from build123d import *

# Parameters (mm, degrees)
SKETCH1_W           = 12.7
SKETCH1_H           = 12.7
BOSS_EXTRUDE1_DEPTH = 2.54
FILLET1_R           = 0.635
SHELL1_START        = 0.635
SHELL1_OUTLINE_W    = 1.905
SHELL1_OUTLINE_H    = 11.43
SHELL1_DEPTH        = 11.43
SKETCH2_R           = 2.54
BOSS_EXTRUDE2_DEPTH = 1.905
BOSS_EXTRUDE4_DEPTH = 0.00254


# Read off the part's stored shape, not the designer's step: Shell1
with BuildPart() as part:
    # Sketch1 → Boss-Extrude1 (new body)
    with BuildSketch(Plane(origin=(0, 0, 0), x_dir=(1, 0, 0), z_dir=(0, 1, 0))):
        with Locations((6.35, 6.35)):
            Rectangle(SKETCH1_W, SKETCH1_H)
    extrude(amount=BOSS_EXTRUDE1_DEPTH)

    # Fillet1
    fillet1_edges = [part.edges().sort_by_distance(p)[0] for p in [
        (0, 1.27, -12.7),
        (12.7, 1.27, -12.7),
        (12.7, 1.27, 0),
        (0, 1.27, 0),
    ]]
    fillet(fillet1_edges, radius=FILLET1_R)

    # Shell1 outline → Shell1 (cut)
    with BuildSketch(Plane.YZ.offset(SHELL1_START)):
        with Locations((0.9525, -6.35)):
            Rectangle(SHELL1_OUTLINE_W, SHELL1_OUTLINE_H)
    extrude(amount=SHELL1_DEPTH, mode=Mode.SUBTRACT)

    # Sketch2 → Boss-Extrude2 (add)
    with BuildSketch(Plane(origin=(0, 1.905, 0), x_dir=(-1, 0, 0), z_dir=(0, -1, 0))):
        with Locations(Location((-6.35, 6.35, 0), (0, 0, 270))):
            Circle(SKETCH2_R)
    extrude(amount=BOSS_EXTRUDE2_DEPTH)

    # Sketch4 → Boss-Extrude4 (add)
    # profile 1 of 2: a face of its own
    with BuildSketch(Plane(origin=(0, 2.54, 0), x_dir=(1, 0, 0), z_dir=(0, 1, 0))):
        with BuildLine():
            Line((6.456138622, 5.974210256), (6.960500601, 5.71853117))
            Line((6.960500601, 5.71853117), (6.407165264, 4.630941026))
            add(Edge.make_bspline(
                [(6.407165264, 4.630941026), (6.439855797, 4.630094651), (6.504245162, 4.628427578), (6.598981047, 4.614954014), (6.689550316, 4.591661453), (6.776866176, 4.560787227), (6.859861273, 4.519322834), (6.939872289, 4.469998775), (7.014829299, 4.40984278), (7.086451002, 4.34319313), (7.151576249, 4.269354895), (7.20814904, 4.190013367), (7.257451228, 4.107098934), (7.295776765, 4.018756598), (7.32669142, 3.926450736), (7.348997703, 3.82981236), (7.361724062, 3.728561626), (7.363478603, 3.659777417), (7.364371795, 3.624761138)],
                knots=[0, 0, 0, 0, 1.013260694, 1.995783107, 2.958651975, 3.908806537, 4.861209129, 5.829647963, 6.817170299, 7.835534541, 8.860094905, 9.863329007, 10.853101798, 11.844815043, 12.84250023, 13.867713965, 14.914507806, 16, 16, 16, 16], degree=3))
            add(Edge.make_bspline(
                [(7.364371795, 3.624761138), (7.3635348, 3.591007569), (7.361880421, 3.524291238), (7.348204784, 3.426301914), (7.326104237, 3.332286889), (7.294518118, 3.242433922), (7.254369605, 3.156303809), (7.205270694, 3.073947091), (7.146814203, 2.995979194), (7.080510488, 2.922814401), (7.008029089, 2.856124152), (6.931629747, 2.796845977), (6.850665063, 2.747879955), (6.766665364, 2.706527002), (6.678084165, 2.675668741), (6.586247088, 2.652376099), (6.490457705, 2.638935234), (6.425438326, 2.63724503), (6.392536859, 2.636389744)],
                knots=[0, 0, 0, 0, 1.049934834, 2.075270938, 3.072134561, 4.05064612, 5.033440221, 6.024524368, 7.028587226, 8.060776465, 9.092543989, 10.090062252, 11.064205434, 12.031961459, 12.998029633, 13.977230324, 14.976426867, 16, 16, 16, 16], degree=3))
            add(Edge.make_bspline(
                [(6.392536859, 2.636389744), (6.358131923, 2.637091632), (6.290479272, 2.6384718), (6.191486511, 2.653926046), (6.096543934, 2.677190259), (6.006185133, 2.710407602), (5.919848194, 2.752703587), (5.838549577, 2.805040616), (5.761604456, 2.866841549), (5.689833178, 2.936715965), (5.625172604, 3.013253826), (5.567500777, 3.092720054), (5.518710337, 3.175239347), (5.479215613, 3.260723478), (5.448400913, 3.348900047), (5.426960167, 3.439936406), (5.412989542, 3.53359108), (5.411351805, 3.597150442), (5.410525641, 3.629213261)],
                knots=[0, 0, 0, 0, 1.063775006, 2.091769615, 3.092589432, 4.084662827, 5.064601646, 6.061867366, 7.070035304, 8.113879863, 9.156342271, 10.166834137, 11.149076039, 12.117706134, 13.076241869, 14.034148791, 15.008317125, 16, 16, 16, 16], degree=3))
            add(Edge.make_bspline(
                [(5.410525641, 3.629213261), (5.41096217, 3.654042164), (5.411837658, 3.703838176), (5.420635786, 3.778404999), (5.434012031, 3.853167552), (5.449516851, 3.916254562), (5.465482147, 3.969601232), (5.481551341, 4.014747076), (5.501465566, 4.064849092), (5.524230475, 4.12003522), (5.550561942, 4.180239071), (5.580322415, 4.245296544), (5.613585986, 4.315700304), (5.637307493, 4.364056786), (5.649668269, 4.389254327)],
                knots=[0, 0, 0, 0, 1.110454016, 2.227089276, 3.35462975, 4.507227546, 5.131400587, 5.845402449, 6.650387134, 7.543487832, 8.516250726, 9.590168902, 10.744287919, 12, 12, 12, 12], degree=3))
            Line((5.649668269, 4.389254327), (6.456138622, 5.974210256))
        make_face()
        with BuildLine():
            add(Edge.make_bspline(
                [(6.379816506, 4.101774359), (6.352472323, 4.100520139), (6.298963346, 4.098065795), (6.222881583, 4.072362713), (6.153512277, 4.032040974), (6.093382105, 3.975885155), (6.043088748, 3.908776745), (6.006131425, 3.832230641), (5.983899541, 3.747268327), (5.981589791, 3.687864094), (5.980397436, 3.657198037)],
                knots=[0, 0, 0, 0, 0.981744412, 1.921144944, 2.858899012, 3.85339082, 4.86292663, 5.863643845, 6.897155691, 8, 8, 8, 8], degree=3))
            add(Edge.make_bspline(
                [(5.980397436, 3.657198037), (5.981809222, 3.626521768), (5.984555239, 3.566854373), (6.007623071, 3.481083067), (6.045392269, 3.402798689), (6.098361161, 3.334800948), (6.160545878, 3.278357558), (6.229501354, 3.236614972), (6.304077387, 3.210971132), (6.35566345, 3.207842243), (6.381724559, 3.206261538)],
                knots=[0, 0, 0, 0, 1.098279937, 2.136227893, 3.159405121, 4.194678092, 5.206500211, 6.154139736, 7.067477469, 8, 8, 8, 8], degree=3))
            add(Edge.make_bspline(
                [(6.381724559, 3.206261538), (6.409248036, 3.207870396), (6.463226355, 3.211025646), (6.54109362, 3.23559044), (6.612225834, 3.276633701), (6.67512047, 3.332896382), (6.729145767, 3.400118178), (6.766525816, 3.478862388), (6.790660084, 3.565252761), (6.79319133, 3.625862449), (6.7945, 3.657198037)],
                knots=[0, 0, 0, 0, 0.96921794, 1.900804717, 2.848419905, 3.844199796, 4.861108892, 5.867439427, 6.897452859, 8, 8, 8, 8], degree=3))
            add(Edge.make_bspline(
                [(6.7945, 3.657198037), (6.793009186, 3.687846189), (6.79012205, 3.747199913), (6.768436237, 3.832560256), (6.729717682, 3.908811323), (6.678286397, 3.976162168), (6.616086864, 4.032292947), (6.543941256, 4.072680703), (6.464383952, 4.098020258), (6.408416654, 4.100504747), (6.379816506, 4.101774359)],
                knots=[0, 0, 0, 0, 1.083229974, 2.097801324, 3.086792542, 4.086858909, 5.079819718, 6.026392613, 6.991456328, 8, 8, 8, 8], degree=3))
        make_face(mode=Mode.SUBTRACT)
    # profile 2 of 2: a face of its own
    with BuildSketch(Plane(origin=(0, 2.54, 0), x_dir=(1, 0, 0), z_dir=(0, 1, 0))):
        Polygon((6.235008013, 10.541), (6.653507612, 10.541), (7.542660256, 8.180102564), (7.026213942, 8.180102564), (6.443621795, 9.726897436), (5.86039363, 8.180102564), (5.344583333, 8.180102564), align=None)
    extrude(amount=BOSS_EXTRUDE4_DEPTH)


solid = part.part
Design review of the part built by this model. Coordinates are the model's own, in mm. A direction names the side the tool comes from. Give positions to 0.01 mm unless a question says otherwise; leave off trailing zeros. Loops run counter-clockwise (first coordinate to the right, second up) from the corner with the lowest first, then second, coordinate; pieces in that order, holes last. Notation, with made-up numbers: M 11.25,17.25 L 58.25,17.25 A23 cw 58.25,50.25 Z; hole C 47.25,30 d1. An arc over 180 degrees is marked long. Answer as a JSON object with one key per item and string values.
Item 1: Mouldability with a two-part tool opening along X and no side actions: class faces 3 (the face through (12.7, 1, -6)), 4 (the face through (0, 1, -6)), 5 (the face through (6, 0, -6)), 6 (the face through (5, 1.905, -9)) as pulls with the +X half, pulls with the -X half, needs draft (parallel to the pull), parting line crosses it, or undercut.
Output values:
{"face 3": "pulls with the +X half", "face 4": "pulls with the -X half", "face 5": "needs draft", "face 6": "undercut"}
Item 2: We need section A-A (y = 1.55). State the section outline as (x, z) points (3 decimals), and give its area (3 significant figures).
Output values:
{"outline": "M 0,-12.065 A0.635 ccw 0.635,-12.7 L 12.065,-12.7 A0.635 ccw 12.7,-12.065 L 12.7,-0.635 A0.635 ccw 12.065,0 L 0.635,0 A0.635 ccw 0,-0.635 Z; C 6.35,-6.35 d5.08; hole M 0.635,-12.065 L 12.065,-12.065 L 12.065,-0.635 L 0.635,-0.635 Z", "area": "50.6 mm2"}
Item 3: We need section C-C (x = 1). State the section outline as (y, z) points (3 decimals), and give its area (3 significant figures).
Output values:
{"outline": "M 0,-12.7 L 2.54,-12.7 L 2.54,0 L 0,0 L 0,-0.635 L 1.905,-0.635 L 1.905,-12.065 L 0,-12.065 Z", "area": "10.5 mm2"}
Item 4: Machinability: for faces 1 (the face through (0.635, 1, -6)), 2 (the face through (6, 2.543, -9)), which of the approach directions +Z, -Z, +X, -X, +Y, -Y give a long, thin tool a straight path to every point of the face, cutting with its end or side? Answer none if there is none.
Output values:
{"face 1": "-Y", "face 2": "+Z, -Z, +X, -X, +Y"}
Item 5: For P1, Ø2, axis at x = 10.5, z = -7.5, coming from the +Y side; P2, Ø2, axis at x = 2.5, z = -7.5, coming from the -Y side (3 decimals), all flat-tipped, find the tip position at first contact; note any pin that passes through.
Output values:
{"P1": "stops at y = 2.54", "P2": "stops at y = 1.905"}
Item 6: Wall thickness on line 1 along X through (y, z) = (1.8, -10) (3 decimals); line 2 along Z through (x, y) = (12, 0.7) (3 decimals); line 3 along X through (y, z) = (0.85, -4.75) (3 decimals): over which ranges is each line inside the solid? List them lowest first.
Output values:
{"line 1": "x = 0 to 0.635, 12.065 to 12.7", "line 2": "z = -12.7 to -12.065, -0.635 to 0", "line 3": "x = 0 to 0.635, 4.377 to 8.323, 12.065 to 12.7"}
Item 7: We need section D-D (z = -6.35). State the section outline as (x, y) points (3 decimals), and give its area (3 significant figures).
Output values:
{"outline": "M 0,0 L 0.635,0 L 0.635,1.905 L 3.81,1.905 L 3.81,0 L 8.89,0 L 8.89,1.905 L 12.065,1.905 L 12.065,0 L 12.7,0 L 12.7,2.54 L 0,2.54 Z", "area": "20.2 mm2"}
Item 8: We need section B-B (z = -1). State the section outline as (x, y) points (3 decimals).
Output values:
{"outline": "M 0,0 L 0.635,0 L 0.635,1.905 L 12.065,1.905 L 12.065,0 L 12.7,0 L 12.7,2.54 L 0,2.54 Z"}
